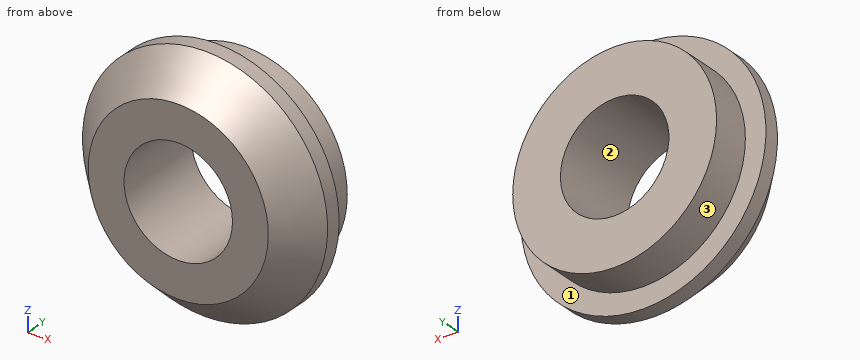
from build123d import *

# Parameters (mm, degrees)
SKETCH1_R               = 9.525
EXTRUDE1_DEPTH          = 7
SKETCH2_R               = 4
EXTRUDE2_DEPTH          = 16.18062087
F_3_8_24_TAPPED_HOLE2_D = 8.4328
SKETCH3_OUTSIDE_W       = 26.618
SKETCH3_OUTSIDE_H       = 26.618
SKETCH3_OUTSIDE_R       = 7.925
EXTRUDE3_DEPTH          = 3


with BuildPart() as part:
    # Sketch1 → Extrude1 (new body)
    with BuildSketch(Plane(origin=(0, 0, 0), x_dir=(1, 0, 0), z_dir=(0, 1, 0))):
        with Locations(Location((0, 0, 0), (0, 0, 270))):
            Circle(SKETCH1_R)
    extrude(amount=EXTRUDE1_DEPTH)

    # Sketch2 → Extrude2 (cut, through all)
    with BuildSketch(Plane(origin=(0, 0, 0), x_dir=(1, 0, 0), z_dir=(0, 1, 0))):
        Circle(SKETCH2_R)
    extrude(amount=EXTRUDE2_DEPTH, mode=Mode.SUBTRACT)

    # 3_8-24 Tapped Hole2 (through all)
    with Locations(Plane(origin=(0, 0, 0), x_dir=(-1, 0, 0), z_dir=(0, -1, 0))):
        with Locations((0, 0)):
            Hole(F_3_8_24_TAPPED_HOLE2_D / 2)

    # Sketch3 outside → Extrude3 (cut)
    with BuildSketch(Plane(origin=(0, 7, 0), x_dir=(1, 0, 0), z_dir=(0, 1, 0))):
        Rectangle(SKETCH3_OUTSIDE_W, SKETCH3_OUTSIDE_H)
        with Locations(Location((0, 0, 0), (0, 0, 270))):
            Circle(SKETCH3_OUTSIDE_R, mode=Mode.SUBTRACT)
    extrude(amount=-EXTRUDE3_DEPTH, mode=Mode.SUBTRACT)

    # Sketch6 → Cut-Revolve1 (revolve, cut)
    with BuildSketch(Plane.XY, mode=Mode.PRIVATE) as cut_revolve1_sk:
        Polygon((-9.525, 2.8), (-7, 0), (-7, -3.811390031), (-11.858524977, -3.811390031), (-11.858524977, 2.8), align=None)
    revolve(cut_revolve1_sk.sketch.rotate(Axis((0, 0, 0), (0, 1, 0)), 270), axis=Axis((0, 0, 0), (0, 1, 0)), mode=Mode.SUBTRACT)


solid = part.part
Here's how the part is built. I have some questions about the finished solid (model axes, mm). Face numbers are marked on the shaded views. Coordinates: 2 decimals unless noted, no trailing zeros. Order: outer loops, then holes, each group sorted by start corner. A loop starts at its lowest first (then second) coordinate and runs counter-clockwise, first axis right, second up. Notation, with made-up numbers: M 21,55 L 46,55 A36 ccw 46,94 Z; hole C 40,52.5 d1. An arc over 180 degrees is marked long. Answer as CSV lines item,"result". Start each with the question number.
1. I need wall thicknesses on line 1 (X direction, y = 4.75, z = 2.75); line 2 (X direction, y = 1, z = -1.5); line 3 (Z direction, x = 6.75, y = 1). Which ranges of each line are inside material? Lowest first, please. Write a range as [from, to].
2. I want a section at C-C, the plane y = 3.25. Write out the boundary of the cut face in (x, z) (3 decimals), and give its area (3 significant figures).
3. I want a section at A-A, the plane z = 0. Write out the boundary of the cut face in (x, y) (3 decimals).
4. For pin 1 (1 mm diameter, centred on x = -4.5, y = 2, fed in from +Z); pin 2 (3 mm diameter, centred on x = -0.5, z = 2, fed in from +Y); pin 3 (4 mm diameter, centred on y = 3.5, z = 7.5, fed in from +X); pin 4 (1 mm diameter, centred on x = 2.5, y = 1.5, fed in from -Z), each with a flat end and sliding along its axis, tell me the tip position at first contact or that it passes through.
5. We'd pull the mould along Z, two halves only. Please class the marked faces 1, 2 and 3: released by +Z, released by -Z, zero draft, split by the parting line, or undercut.
6. I want a section at B-B, the plane x = 0. Write out the boundary of the cut face in (y, z) (3 decimals).
Recorded:
1,line 1,"x = [-7.43, -3.2], [3.2, 7.43]"
1,line 2,"x = [-7.76, -3.94], [3.94, 7.76]"
1,line 3,"z = [-4.11, 4.11]"
2,outline,"C 0,0 d19.05; hole C 0,0 d8.433"
2,area,"229 mm2"
3,outline,"M -9.525,2.8 L -7,0 L -4.216,0 L -4.216,7 L -7.925,7 L -7.925,4 L -9.525,4 Z; M 4.216,0 L 7,0 L 9.525,2.8 L 9.525,4 L 7.925,4 L 7.925,7 L 4.216,7 Z"
4,pin 1,"stops at z = 8.15"
4,pin 2,"passes through"
4,pin 3,"stops at x = 7.78"
4,pin 4,"stops at z = -8.46"
5,face 1,"zero draft"
5,face 2,"undercut"
5,face 3,"split by the parting line"
6,outline,"M 0,-7 L 2.8,-9.525 L 4,-9.525 L 4,-7.925 L 7,-7.925 L 7,-4.216 L 0,-4.216 Z; M 0,4.216 L 7,4.216 L 7,7.925 L 4,7.925 L 4,9.525 L 2.8,9.525 L 0,7 Z"
